Could you check a few things on this model? Use its own coordinates, in mm. Give positions to 0.01 mm unless a question says otherwise; leave off trailing zeros. Write each loop counter-clockwise with the first axis right and the second up, starting at its lowest first coordinate (ties: lowest second). Pieces come first, ordered by that corner, then holes. Notation, with made-up numbers: M -33,-18 L 4,-18 A10 cw 4,-12 Z; hole C 46.5,-23 d7. An arc over 180 degrees is marked long. One line per item, written item: value.
```python
from build123d import *

# Parameters (mm, degrees)
SKETCH1_R           = 8
SKETCH1_R_2         = 4
BOSS_EXTRUDE1_DEPTH = 5
FILLET1_R           = 0.2
SKETCH2_R           = 7
SKETCH2_R_2         = 5
CUT_EXTRUDE1_DEPTH  = 0.1
CUT_EXTRUDE2_START  = -0.1
SKETCH3_R           = 7
SKETCH3_R_2         = 5
CUT_EXTRUDE2_DEPTH  = 0.1


with BuildPart() as part:
    # Sketch1 → Boss-Extrude1 (new body)
    with BuildSketch(Plane(origin=(0, 0, 0), x_dir=(1, 0, 0), z_dir=(0, 1, 0))):
        with Locations(Location((0, 0, 0), (0, 0, 270))):
            Circle(SKETCH1_R)
        with Locations(Location((0, 0, 0), (0, 0, 270))):
            Circle(SKETCH1_R_2, mode=Mode.SUBTRACT)
    extrude(amount=BOSS_EXTRUDE1_DEPTH)

    # Fillet1
    fillet1_edges = [part.edges().sort_by_distance(p)[0] for p in [
        (0, 0, -8),
        (0, 5, -8),
        (0, 0, -4),
        (0, 5, -4),
    ]]
    fillet(fillet1_edges, radius=FILLET1_R)

    # Sketch2 → Cut-Extrude1 (cut)
    with BuildSketch(Plane(origin=(0, 5, 0), x_dir=(1, 0, 0), z_dir=(0, 1, 0))):
        with Locations(Location((0, 0, 0), (0, 0, 270))):
            Circle(SKETCH2_R)
        with Locations(Location((0, 0, 0), (0, 0, 270))):
            Circle(SKETCH2_R_2, mode=Mode.SUBTRACT)
    extrude(amount=-CUT_EXTRUDE1_DEPTH, mode=Mode.SUBTRACT)

    # Sketch3 → Cut-Extrude2 (cut)
    with BuildSketch(Plane.XZ.offset(CUT_EXTRUDE2_START)):
        with Locations(Location((0, 0, 0), (0, 0, 90))):
            Circle(SKETCH3_R)
        with Locations(Location((0, 0, 0), (0, 0, 90))):
            Circle(SKETCH3_R_2, mode=Mode.SUBTRACT)
    extrude(amount=CUT_EXTRUDE2_DEPTH, mode=Mode.SUBTRACT)


solid = part.part
```
1) I'm going to push a flat-ended pin straight in: pin 1 (3 mm diameter, centred on y = 2.5, z = 6, fed in from +X). Where does the tip first touch, or does it pass through?
Outcome:
pin 1: stops at x = 6.61
2) Please list where these lines run through material, in increasing order: L1, parallel to X at y = 3.05, z = 0; L2, parallel to X at y = 4.95, z = 0; L3, parallel to Y at x = 6.75, z = 1. Write a range as from..to.
Outcome:
L1: x = -8..-4, 4..8
L2: x = -7.93..-7, -5..-4.07, 4.07..5, 7..7.93
L3: y = 0.1..4.9
3) If we section it at C-C, the plane y = 1.15: Write out the boundary of the cut face in (x, z).
Outcome:
outline: C 0,0 d16; hole C 0,0 d8
4) We'd pull the mould along X, two halves only. Please class faces 1 (the face through (4, 0, -6)), 2 (the face through (-5, 0.1, -2)), 3 (the face through (5, 4.9, -2)), 4 (the face through (-7.81, 2.47, -1.73)): pulls with the +X half, pulls with the -X half, needs draft (parallel to the pull), parting line crosses it, or undercut.
Outcome:
face 1: needs draft
face 2: undercut
face 3: undercut
face 4: parting line crosses it
